```python
from build123d import *

# Parameters (mm, degrees)
SKETCH2_W           = 25.1
SKETCH2_H           = 57.2
SKETCH2_R           = 1.335
BOSS_EXTRUDE1_DEPTH = 3
BOSS_EXTRUDE2_DEPTH = 6
FILLET1_R           = 2


with BuildPart() as part:
    # Sketch2 → Boss-Extrude1 (new body)
    with BuildSketch(Plane(origin=(0, 0, 0), x_dir=(1, 0, 0), z_dir=(0, 1, 0))):
        with Locations((0, 28.6)):
            Rectangle(SKETCH2_W, SKETCH2_H)
        with Locations((0, 24.5)):
            Circle(SKETCH2_R, mode=Mode.SUBTRACT)
    boss_extrude1 = extrude(amount=BOSS_EXTRUDE1_DEPTH)

    # Sketch4 → Boss-Extrude2 (add)
    with BuildSketch(Plane(origin=(0, 0, -57.2), x_dir=(-1, 0, 0), z_dir=(0, 0, -1))):
        Polygon((12.55, 0), (-12.55, 0), (-12.55, -10.65), (-7.55, -10.65), (-7.55, -5.65), (7.55, -5.65), (7.55, -10.65), (12.55, -10.65), align=None)
    boss_extrude2 = extrude(amount=-BOSS_EXTRUDE2_DEPTH)

    # Mirror1: Boss-Extrude1, Boss-Extrude2 across plane
    add(boss_extrude1.mirror(Plane.XY))
    add(boss_extrude2.mirror(Plane.XY))

    # Fillet1
    fillet1_edges = [part.edges().sort_by_distance(p)[0] for p in [
        (0, 3, -57.2),
        (0, 3, 57.2),
    ]]
    fillet(fillet1_edges, radius=FILLET1_R)


solid = part.part
```
The model under review builds one solid part; all positions refer to its coordinate system, in mm. A direction names the side the tool comes from. Coordinates: 2 decimals unless noted, no trailing zeros. Write each loop counter-clockwise with the first axis right and the second up, starting at its lowest first coordinate (ties: lowest second). Pieces come first, ordered by that corner, then holes.
1) We need section C-C on y = -6.75. State the section outline as (x, z) points.
2) Machinability: for faces 4 (the face through (-10, -10.65, 54)), 5 (the face through (0, -4, 51.2)), 6 (the face through (7.55, -8, -54)), which of the approach directions +Z, -Z, +X, -X, +Y, -Y give a long, thin tool a straight path to every point of the face, cutting with its end or side? Answer none if there is none.
3) We need section A-A on z = 24.5. State the section outline as (x, y) points (3 decimals).
4) To check wall thickness, follow probe 1 along Z at (x, y) = (0, 1.25) (3 decimals); probe 2 along Z at (x, y) = (-11, -1); probe 3 along Z at (x, y) = (0, 1.9) (3 decimals). State the ranges of each line that lie inside material, in increasing order.
5) The part is to be moulded in two halves that separate along Z. For faces 1 (the face through (0, 3, 1)), 2 (the face through (0.18, 2.4, -56.63)), 3 (the face through (-0.3, 1.5, -23.2)), say which applies: pulls with the +Z half, pulls with the -Z half, needs draft (parallel to the pull), parting line crosses it, or undercut.
6) We need section D-D on x = -5.75. State the section outline as (y, z) points.
7) Clearance check with flat-ended pins moving along their axes: pin 1 Ø4.5 at (x, z) = (0, 24.5) entering from -Y; pin 2 Ø3 at (x, z) = (3.5, 52.5) entering from -Y. State where each tip first meets the part, or that it passes through.
8) We need section B-B on x = 0. State the section outline as (y, z) points (3 decimals).
Answer list:
1. outline: (-12.55, -57.2) - (-7.55, -57.2) - (-7.55, -51.2) - (-12.55, -51.2) - close; (-12.55, 51.2) - (-7.55, 51.2) - (-7.55, 57.2) - (-12.55, 57.2) - close; (7.55, -57.2) - (12.55, -57.2) - (12.55, -51.2) - (7.55, -51.2) - close; (7.55, 51.2) - (12.55, 51.2) - (12.55, 57.2) - (7.55, 57.2) - close
2. face 4: +Z, -Z, +X, -X, -Y
2. face 5: +X, -X, -Y
2. face 6: +Z, -Z, -Y
3. outline: (-12.55, 0) - (-1.335, 0) - (-1.335, 3) - (-12.55, 3) - close; (1.335, 0) - (12.55, 0) - (12.55, 3) - (1.335, 3) - close
4. probe 1: z = -57.184 to -25.835, -23.165 to 23.165, 25.835 to 57.184
4. probe 2: z = -57.2 to -51.2, 51.2 to 57.2
4. probe 3: z = -56.986 to -25.835, -23.165 to 23.165, 25.835 to 56.986
5. face 1: needs draft
5. face 2: pulls with the -Z half
5. face 3: undercut
6. outline: (-5.65, -57.2) - (1, -57.2) arc R2 ccw to (3, -55.2) - (3, 55.2) arc R2 ccw to (1, 57.2) - (-5.65, 57.2) - (-5.65, 51.2) - (0, 51.2) - (0, -51.2) - (-5.65, -51.2) - close
7. pin 1: stops at y = 0
7. pin 2: stops at y = -5.65
8. outline: (-5.65, -57.2) - (1, -57.2) arc R2 ccw to (3, -55.2) - (3, -25.835) - (0, -25.835) - (0, -51.2) - (-5.65, -51.2) - close; (-5.65, 51.2) - (0, 51.2) - (0, 25.835) - (3, 25.835) - (3, 55.2) arc R2 ccw to (1, 57.2) - (-5.65, 57.2) - close; (0, -23.165) - (3, -23.165) - (3, 23.165) - (0, 23.165) - close
